```python
from build123d import *

# Parameters (mm, degrees)
F2_SIZE = 1


with BuildPart() as f1:
    # F0 (on Right) → F1 (revolve)
    with BuildSketch(Plane.YZ):
        Polygon((0, 12), (0, 9), (44, 9), (44, 12.25), (37, 12.25), (37, 15), (12.1, 15), (12.1, 12), (11.1, 12), (9.6, 10.5), (8.1, 12), align=None)
    revolve(axis=Axis((0, 15.313713, 0), (0, 1, 0)))

    # F2
    f2_edges = [f1.edges().sort_by_distance(p)[0] for p in [
        (0, 0, -12),
    ]]
    chamfer(f2_edges, length=F2_SIZE)


solid = f1.part
```
For this review, take the finished solid that the model builds, in its own axes (mm). A direction names the side the tool comes from. Give positions to 0.01 mm unless a question says otherwise; leave off trailing zeros. Write each loop counter-clockwise with the first axis right and the second up, starting at its lowest first coordinate (ties: lowest second). Pieces come first, ordered by that corner, then holes.
Item 1: Wall thickness on probe 1 along X at (y, z) = (22, 0); probe 2 along Y at (x, z) = (13.25, 5.25); probe 3 along X at (y, z) = (25.5, 8.25): over which ranges is each line inside the solid? List them lowest first.
Item 2: Take a section at C-C (y = 15). Give the boundary of the cut face in (x, z).
Item 3: Take a section at A-A (z = 0). Give the boundary of the cut face in (x, y), and give its area (3 significant figures).
Item 4: Take a section at B-B (x = 0). Give the boundary of the cut face in (y, z), and give its area (3 significant figures).
Item 5: Insertion check: P1, Ø1.5, axis at x = 8, y = 17.5, coming from the -Z side; P2, Ø3, axis at x = -7, z = -1, coming from the -Y side; P3, Ø10, axis at x = -7.5, y = 13.5, coming from the -Z side; P4, Ø6, axis at y = 24, z = 11.5, coming from the -X side. Each pin has a flat end and moves straight along its axis. Give the tip position at first contact, or say it passes through.
Item 6: The part is to be moulded in two halves that separate along Z. For faces 1 (the face through (0.53, 11.59, -11.99)), 2 (the face through (-9, 0, 2)), 3 (the face through (8.923, 22.308, -1.172)), say which applies: +Z half, -Z half, draft (parallel to the pull), parting line (faces both ways), or undercut.
Item 7: Machinability: for faces 4 (the face through (0.66, 24.376, -14.985)), 5 (the face through (0.53, 4.5, -11.99)), 6 (the face through (-11, 37, 6)), which of the approach directions +Z, -Z, +X, -X, +Y, -Y give a long, thin tool a straight path to every point of the face, cutting with its end or side? Answer none if there is none.
Established:
1. probe 1: x = -15 to -9, 9 to 15
1. probe 2: y = 12.1 to 37
1. probe 3: x = -12.53 to -3.6, 3.6 to 12.53
2. outline: circle Ø30 at (0, 0); hole circle Ø18 at (0, 0)
3. outline: (-15, 12.1) - (-12, 12.1) - (-12, 11.1) - (-10.5, 9.6) - (-12, 8.1) - (-12, 1) - (-11, 0) - (-9, 0) - (-9, 44) - (-12.25, 44) - (-12.25, 37) - (-15, 37) - close; (9, 0) - (11, 0) - (12, 1) - (12, 8.1) - (10.5, 9.6) - (12, 11.1) - (12, 12.1) - (15, 12.1) - (15, 37) - (12.25, 37) - (12.25, 44) - (9, 44) - close
3. area: 411 mm2
4. outline: (0, -11) - (1, -12) - (8.1, -12) - (9.6, -10.5) - (11.1, -12) - (12.1, -12) - (12.1, -15) - (37, -15) - (37, -12.25) - (44, -12.25) - (44, -9) - (0, -9) - close; (0, 9) - (44, 9) - (44, 12.25) - (37, 12.25) - (37, 15) - (12.1, 15) - (12.1, 12) - (11.1, 12) - (9.6, 10.5) - (8.1, 12) - (1, 12) - (0, 11) - close
4. area: 411 mm2
5. P1: stops at z = -13.13
5. P2: passes through
5. P3: stops at z = -14.79
5. P4: stops at x = -12.36
6. face 1: parting line
6. face 2: draft
6. face 3: undercut
7. face 4: +Y, -Y
7. face 5: -Y
7. face 6: +Y
